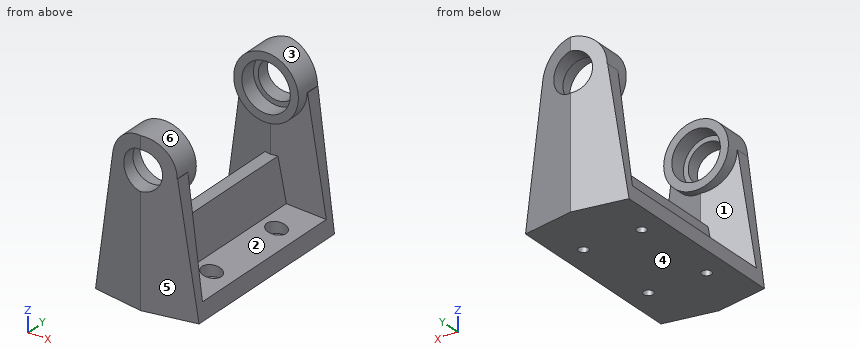
Autodesk Fusion 360 part; units mm, degrees
sketch "草图1" plane through (0, 0, 0) normal (0, 1, 0) x (1, 0, 0)
  circle A0 centre (0, 0) radius 10
  circle A1 centre (0, 0) radius 7.5
  circle A2 centre (0, 0) radius 6
  line L0 (-9.8932, -1.4573) -> (-16, 40)
  line L1 (-16, 40) -> (16, 40)
  line L2 (16, 40) -> (9.8932, -1.4573)
  line L3 (0, -55) -> (0, 135) construction
  line L4 (-15.2635, 35) -> (-4.3042, 33.0676)
  line L5 (-4.3042, 33.0676) -> (-2, 20)
  line L6 (-2, 20) -> (2, 20)
  line L7 (2, 20) -> (4.3042, 33.0676)
  line L8 (4.3042, 33.0676) -> (15.2635, 35)
  dimension "d1" = 32
  dimension "d2" = 12
  dimension "d3" = 15
  dimension "d4" = 20
  dimension "d5" = 40
  dimension "d6" = 4
  dimension "d7" = 5
  dimension "d8" = 20
  dimension "d9" = 20
  dimension "d10" = 10
extrude "拉伸1" add sketch "草图1" along normal blind 64 contours L0 L1 L2 L4 L5 L6 L7 L8 makes body 1
extrude "拉伸2" add sketch "草图1" along normal blind 8 separate body contours A0 L0 L2 L4 L5 L6 L7 L8 makes body 2
extrude "拉伸3" add sketch "草图1" along normal blind 10 separate body contours A0 makes body 3
extrude "拉伸4" add sketch "草图1" along normal blind 5 contours A1 bodies 3
copy_body "复制和粘贴实体1" bodies 2 makes body 4
move_body "移动1" bodies 4 to x (1, 0, 0) y (0, 1, 0) z (0, 0, 1) at (0, 14, 0)
move_body "移动2" bodies 4 to x (1, 0, 0) y (0, 1, 0) z (0, 0, 1) at (0, 42, 0)
sketch "草图2" plane through (0, 0, 0) normal (0, 0, 1) x (1, 0, 0)
  line L0 (0, 60) -> (0, -25) construction
  line L1 (0, 0) -> (16, 2.8212)
  line L2 (16, 2.8212) -> (16, 5.1788)
  line L3 (16, 5.1788) -> (0, 8)
  line L4 (0, 8) -> (-16, 5.1788)
  line L5 (-16, 5.1788) -> (-16, 2.8212)
  line L6 (-16, 2.8212) -> (0, 0)
  line L7 (0, 56) -> (16, 58.8212)
  line L8 (16, 58.8212) -> (16, 61.1788)
  line L9 (16, 61.1788) -> (0, 64)
  line L10 (0, 64) -> (-16, 61.1788)
  line L11 (-16, 61.1788) -> (-16, 58.8212)
  line L12 (-16, 58.8212) -> (0, 56)
  line L13 (10, 0) -> (-10, 0)
  line L14 (0, 8) -> (15, 8) construction
  line L15 (0, 56) -> (15, 56) construction
  line L16 (0, 64) -> (14, 64) construction
  line L17 (0, 64) -> (-16, 64)
  line L18 (-16, 64) -> (-16, 0)
  line L19 (-16, 0) -> (16, 0)
  line L20 (16, 0) -> (16, 64)
  line L21 (16, 64) -> (0, 64)
  dimension "d19" = 64
  dimension "d20" = 10
  dimension "d21" = 48
  dimension "d22" = 10
  dimension "d23" = 10
  dimension "d24" = 32
  dimension "d25" = 32
extrude "拉伸5" cut sketch "草图2" against normal blind 160 contours L1 L2 L3 L4 L5 L6 L18 L20 | L7 L8 L9 L10 L11 L12 L18 L20 keep common part bodies 2 4
extrude "拉伸6" cut sketch "草图2" against normal blind 105 contours L1 L2 L3 L4 L5 L6 L18 L20 | L3 L4 L7 L12 L18 L20 | L7 L8 L9 L10 L11 L12 L18 L20 keep common part bodies 1
extrude "拉伸7" cut sketch "草图2" along normal mid plane 30 contours L6 L13 L18 L19 | L1 L13 L19 L20 bodies 3
copy_body "复制和粘贴实体2" bodies 3 makes body 5
move_body "移动3" bodies 5 to x (1, 0, 0) y (0, -1, 0) z (0, 0, -1) at (0, 50, 0)
move_body "移动4" bodies 5 to x (1, 0, 0) y (0, 1, 0) z (0, 0, 1) at (0, 14, 0)
combine "合并1" operation add target body 1 tool bodies 2 3 5 4
sketch "草图3" plane through (0, 0, 0) normal (0, 0, 1) x (1, 0, 0)
  line L0 (16, 0) -> (-16, 0)
  line L1 (-16, 0) -> (-16, 64)
  line L2 (-16, 64) -> (16, 64)
  line L3 (16, 64) -> (16, 0)
  line L4 (0, -10) -> (0, 70) construction
  circle A0 centre (9, 18) radius 3
  circle A1 centre (9, 18) radius 1.5
  circle A2 centre (-9, 18) radius 3
  circle A3 centre (-9, 18) radius 1.5
  circle A4 centre (9, 46) radius 3
  circle A5 centre (9, 46) radius 1.5
  circle A6 centre (-9, 46) radius 3
  circle A7 centre (-9, 46) radius 1.5
  line L5 (16, 32) -> (-16, 32) construction
  dimension "d32" = 32
  dimension "d33" = 64
  dimension "d34" = 6
  dimension "d35" = 3
  dimension "d36" = 28
  dimension "d37" = 28
  dimension "d38" = 18
extrude "拉伸8" cut sketch "草图3" against normal through all contours A1 | A3 | A5 | A7 bodies 1
extrude "拉伸9" cut sketch "草图3" against normal blind 37 contours A0 | A2 | A4 | A6 bodies 1
Geometry check sheet. Reference: the model listing, model coordinates, mm. Face numbers are marked on the shaded views. A direction names the side the tool comes from. Round coordinates to 2 decimals unless told otherwise and drop trailing zeros. Loops run counter-clockwise (first coordinate to the right, second up) from the corner with the lowest first, then second, coordinate; pieces in that order, holes last. Notation, with made-up numbers: M 28.5,3 L 79.5,3 A28 cw 79.5,29 Z; hole C 6.5,58.25 d3. An arc over 180 degrees is marked long. Return JSON: item names as keys, results as strings. Group by question number.
(1) Mould release check, pull along Z, two halves, no side actions. Record for the marked faces 4, 5 and 6: pulls with the +Z half, pulls with the -Z half, needs draft (parallel to the pull), parting line crosses it, or undercut.
(2) Section check A-A, the plane z = -11. Enter the section's corners in (x, y), and give its area (3 significant figures).
(3) Go/stop test with flat-tipped pins: pin 1 (7 mm diameter, centred on x = 0, z = 0, fed in from +Y) (3 decimals); pin 2 (4 mm diameter, centred on x = -12.5, z = -21, fed in from -Y); pin 3 (1 mm diameter, centred on x = -7, z = -34, fed in from -Y); pin 4 (7.5 mm diameter, centred on x = -3, z = -0.5, fed in from -Y). Record where each tip stops, or that it passes through.
(4) Section check B-B, the plane x = -9. Enter the section's corners in (y, z), and give its area (3 significant figures).
(5) Scan lines: line 1 along Y through (x, z) = (8, -12); line 2 along Z through (x, y) = (0, 57.05); line 3 along Z through (x, y) = (0, 60.15). Record each from-to range of solid material in increasing order. Write a range as [from, to].
(6) Section check D-D, the plane y = 26.5. Enter the section's corners in (x, z), and give its area (3 significant figures).
(7) Set-up check for the marked faces 1, 2 and 3: record each of +Z, -Z, +X, -X, +Y, -Y from which the full face is reachable in a straight line by a thin tool's end or side.
(8) Section check C-C, the plane y = 18. Enter the section's corners in (x, z).
Data:
{
 "1": {"face 4": "pulls with the -Z half", "face 5": "needs draft", "face 6": "undercut"},
 "2": {"outline": "M -11.73,2.07 L 0,0 L 11.73,2.07 L 11.73,5.93 L 0,8 L -11.73,5.93 Z; M -11.73,58.07 L 0,56 L 11.73,58.07 L 11.73,61.93 L 0,64 L -11.73,61.93 Z", "area": "278 mm²"},
 "3": {"pin 1": "through", "pin 2": "y = 1.85", "pin 3": "y = 1.15", "pin 4": "y = 0.8"},
 "4": {"outline": "M 1.59,-40 L 16.5,-40 L 16.5,-37 L 15,-37 L 15,-33.9 L 6.41,-33.9 L 6.41,-4.36 L 10,-4.36 L 10,4.36 L 1.59,4.36 Z; M 19.5,-40 L 44.5,-40 L 44.5,-37 L 43,-37 L 43,-33.9 L 21,-33.9 L 21,-37 L 19.5,-37 Z; M 47.5,-40 L 62.41,-40 L 62.41,4.36 L 54,4.36 L 54,-4.36 L 57.59,-4.36 L 57.59,-33.9 L 49,-33.9 L 49,-37 L 47.5,-37 Z", "area": "748 mm²"},
 "5": {"line 1": "[1.41, 6.59], [57.41, 62.59]", "line 2": "[-40, -7.5], [7.5, 10]", "line 3": "[-40, -6], [6, 10]"},
 "6": {"outline": "M -16,-40 L 16,-40 L 15.26,-35 L 4.3,-33.07 L 2,-20 L -2,-20 L -4.3,-33.07 L -15.26,-35 Z", "area": "277 mm²"},
 "7": {"face 1": "-X", "face 2": "+X", "face 3": "none"},
 "8": {"outline": "M -16,-40 L -10.5,-40 L -10.5,-37 L -12,-37 L -12,-34.42 L -15.26,-35 Z; M -7.5,-40 L 7.5,-40 L 7.5,-37 L 6,-37 L 6,-33.37 L 4.3,-33.07 L 2,-20 L -2,-20 L -4.3,-33.07 L -6,-33.37 L -6,-37 L -7.5,-37 Z; M 10.5,-40 L 16,-40 L 15.26,-35 L 12,-34.42 L 12,-37 L 10.5,-37 Z"}
}
